from build123d import *

# Parameters (mm, degrees)
F0_R     = 5
F0_W     = 5.4
F0_H     = 5.4
F1_DEPTH = 3
F2_R     = 0.6


with BuildPart() as f1:
    # F0 (on Top) → F1 (new body)
    with BuildSketch(Plane.XY):
        Circle(F0_R)
        Rectangle(F0_W, F0_H, mode=Mode.SUBTRACT)
    extrude(amount=F1_DEPTH)

    # F2
    f2_edges = [f1.edges().sort_by_distance(p)[0] for p in [
        (5, 0, 1.5),
        (-5, 0, 0),
        (-5, 0, 3),
    ]]
    fillet(f2_edges, radius=F2_R)


solid = f1.part
Design review of the part built by this model. Coordinates are the model's own, in mm. A direction names the side the tool comes from. Give positions to 0.01 mm unless a question says otherwise; leave off trailing zeros. Loops run counter-clockwise (first coordinate to the right, second up) from the corner with the lowest first, then second, coordinate; pieces in that order, holes last. Notation, with made-up numbers: M -30,22.5 L 19,22.5 A19 cw 19,45.5 Z; hole C -5.75,29 d8. An arc over 180 degrees is marked long. Answer as a JSON object with one key per item and string values.
Item 1: We need section A-A (x = 0). State the section outline as (y, z) points.
Output values:
{"outline": "M -5,0.6 A0.6 ccw -4.4,0 L -2.7,0 L -2.7,3 L -4.4,3 A0.6 ccw -5,2.4 Z; M 2.7,0 L 4.4,0 A0.6 ccw 5,0.6 L 5,2.4 A0.6 ccw 4.4,3 L 2.7,3 Z"}
Item 2: We need section D-D (z = 2.8). State the section outline as (x, y) points.
Output values:
{"outline": "C 0,0 d9.69; hole M -2.7,-2.7 L 2.7,-2.7 L 2.7,2.7 L -2.7,2.7 Z"}
Item 3: Mouldability with a two-part tool opening along X and no side actions: class faces 3 (the face through (0, 2.7, 1)), 4 (the face through (0, -3, 3)), 5 (the face through (-2.7, 0, 1)), 6 (the face through (-1.08, -4.88, 1.49)) as pulls with the +X half, pulls with the -X half, needs draft (parallel to the pull), parting line crosses it, or undercut.
Output values:
{"face 3": "undercut", "face 4": "needs draft", "face 5": "undercut", "face 6": "parting line crosses it"}
Item 4: Wall thickness on line 1 along Y through (x, z) = (-1.75, 1.55); line 2 along Y through (x, z) = (2, 1.3); line 3 along X through (y, z) = (-1.5, 0.6): over which ranges is each line inside the solid? List them lowest first.
Output values:
{"line 1": "y = -4.68 to -2.7, 2.7 to 4.68", "line 2": "y = -4.58 to -2.7, 2.7 to 4.58", "line 3": "x = -4.77 to -2.7, 2.7 to 4.77"}
Item 5: We need section C-C (z = 1.3). State the section outline as (x, y) points, and give its area (3 significant figures).
Output values:
{"outline": "C 0,0 d10; hole M -2.7,-2.7 L 2.7,-2.7 L 2.7,2.7 L -2.7,2.7 Z", "area": "49.4 mm2"}
Item 6: For P1, Ø1.5, axis at x = -1, z = 2, coming from the -Y side, flat-tipped, find the tip position at first contact; note if it passes through.
Output values:
{"P1": "stops at y = -4.99"}
Item 7: Machinability: for faces 1 (the face through (0, -3, 0)), 2 (the face through (0, -2.7, 1)), which of the approach directions +Z, -Z, +X, -X, +Y, -Y give a long, thin tool a straight path to every point of the face, cutting with its end or side? Answer none if there is none.
Output values:
{"face 1": "-Z, +X, -X, +Y, -Y", "face 2": "+Z, -Z"}
